Source: CAD feature listing. Evaluate the final solid. Frame: model axes, mm. A direction names the side the tool comes from. Coordinates: 2 decimals unless noted, no trailing zeros. Loops run counter-clockwise (first coordinate to the right, second up) from the corner with the lowest first, then second, coordinate; pieces in that order, holes last.
Item 1: Section query D-D, the plane y = 6.5. State how many separate pieces and enclosed holes the cut face has, then the cut area to 3 significant figures.
Item 2: Line query: probe 1 along X at (y, z) = (2, 0); probe 2 along X at (y, z) = (9.5, 10); probe 3 along X at (y, z) = (2.25, -1). Output: solid intervals per line, ascending.
Item 3: Pin query (flat end, axial travel): pin 1 Ø4 at (y, z) = (8, -4) entering from +X; pin 2 Ø2.5 at (x, z) = (-11.31, 11.31) entering from +Y; pin 3 Ø4 at (x, z) = (-11.31, -11.31) entering from +Y; pin 4 Ø1 at (x, y) = (-9, 1.5) entering from -Z. Return the tip coordinate at first contact, or that it passes through.
Item 4: Pull-direction query (Z, two-part tool) for faces 3 (the cylindrical face through (-12.924, 5.07, -11.671)), 4 (the cylindrical face through (-26.36, 4.93, -5.85)), 5 (the flat face through (0, 0, 6)); classes: +Z half, -Z half, draft (parallel to the pull), parting line (faces both ways), or undercut.
Item 5: Section query A-A, the plane z = 0. Return the cut outline in (x, y).
Item 6: Reachability of faces 1 (the flat face through (-2, 5, 0)), 2 (the flat face through (0, 10, 6)) from +Z, -Z, +X, -X, +Y, -Y: full face, straight path, thin tool, end or side. Return the list, or none.
Item 7: Section query B-B, the plane x = -16. Return the cut outline in (y, z), then the cut area to 3 significant figures.
Item 8: Section query C-C, the plane z = -16. Return the cut outline in (x, y), then the cut area to 3 significant figures.
```python
from build123d import *

# Parameters (mm, degrees)
SKETCH1_R           = 27
BOSS_EXTRUDE1_DEPTH = 10
CUT_EXTRUDE1_DEPTH  = 10
SKETCH3_R           = 1.65
CUT_EXTRUDE2_DEPTH  = 10


with BuildPart() as part:
    # Sketch1 → Boss-Extrude1 (new body)
    with BuildSketch(Plane(origin=(0, 0, 0), x_dir=(1, 0, 0), z_dir=(0, 1, 0))):
        with Locations(Location((0, 0, 0), (0, 0, 270))):
            Circle(SKETCH1_R)
    extrude(amount=BOSS_EXTRUDE1_DEPTH)

    # Sketch2 → Cut-Extrude1 (cut)
    with BuildSketch(Plane(origin=(0, 10, 0), x_dir=(1, 0, 0), z_dir=(0, 1, 0))):
        with BuildLine():
            Line((-2, 4.582575695), (-2, -4.582575695))
            ThreePointArc((-2, -4.582575695), (0, -5), (2, -4.582575695))
            Line((2, -4.582575695), (2, 4.582575695))
            ThreePointArc((2, 4.582575695), (0, 5), (-2, 4.582575695))
        make_face()
    extrude(amount=-CUT_EXTRUDE1_DEPTH, mode=Mode.SUBTRACT)

    # Sketch3 → Cut-Extrude2 (cut)
    with BuildSketch(Plane(origin=(0, 10, 0), x_dir=(1, 0, 0), z_dir=(0, 1, 0))):
        with Locations(Location((16, 0, 0), (0, 0, 270))):
            Circle(SKETCH3_R)
        with Locations(Location((11.313708499, -11.313708499, 0), (0, 0, 270))):
            Circle(SKETCH3_R)
        with Locations(Location((0, -16, 0), (0, 0, 270))):
            Circle(SKETCH3_R)
        with Locations(Location((-11.313708499, -11.313708499, 0), (0, 0, 270))):
            Circle(SKETCH3_R)
        with Locations(Location((-16, 0, 0), (0, 0, 270))):
            Circle(SKETCH3_R)
        with Locations(Location((-11.313708499, 11.313708499, 0), (0, 0, 270))):
            Circle(SKETCH3_R)
        with Locations(Location((0, 16, 0), (0, 0, 270))):
            Circle(SKETCH3_R)
        with Locations(Location((11.313708499, 11.313708499, 0), (0, 0, 270))):
            Circle(SKETCH3_R)
    extrude(amount=-CUT_EXTRUDE2_DEPTH, mode=Mode.SUBTRACT)


solid = part.part
```
Verdict:
1. separate pieces: 1
1. enclosed holes: 9
1. area: 2,180 mm2
2. probe 1: x = -27 to -17.65, -14.35 to -2, 2 to 14.35, 17.65 to 27
2. probe 2: x = -25.08 to -12.31, -10.32 to 10.32, 12.31 to 25.08
2. probe 3: x = -26.98 to -17.31, -14.69 to -2, 2 to 14.69, 17.31 to 26.98
3. pin 1: stops at x = 26.93
3. pin 2: passes through
3. pin 3: stops at y = 10
3. pin 4: stops at z = -25.63
4. face 3: undercut
4. face 4: parting line
4. face 5: draft
5. outline: (-27, 0) - (-17.65, 0) - (-17.65, 10) - (-27, 10) - close; (-14.35, 0) - (-2, 0) - (-2, 10) - (-14.35, 10) - close; (2, 0) - (14.35, 0) - (14.35, 10) - (2, 10) - close; (17.65, 0) - (27, 0) - (27, 10) - (17.65, 10) - close
6. face 1: +Y, -Y
6. face 2: +Z, -Z, +X, -X, +Y
7. outline: (0, -21.75) - (10, -21.75) - (10, -1.65) - (0, -1.65) - close; (0, 1.65) - (10, 1.65) - (10, 21.75) - (0, 21.75) - close
7. area: 402 mm2
8. outline: (-21.75, 0) - (-1.65, 0) - (-1.65, 10) - (-21.75, 10) - close; (1.65, 0) - (21.75, 0) - (21.75, 10) - (1.65, 10) - close
8. area: 402 mm2
